Read the model definition and answer for the solid it produces. Units are mm, in the model's axes. Face numbers are marked on the shaded views. A direction names the side the tool comes from. Give positions to 0.01 mm unless a question says otherwise; leave off trailing zeros. Order: outer loops, then holes, each group sorted by start corner. A loop starts at its lowest first (then second) coordinate and runs counter-clockwise, first axis right, second up. Notation, with made-up numbers: M 50,66.5 L 103,66.5 A5 ccw 103,71.5 Z; hole C 54,74.5 d2. An arc over 180 degrees is marked long. One line per item, written item: value.
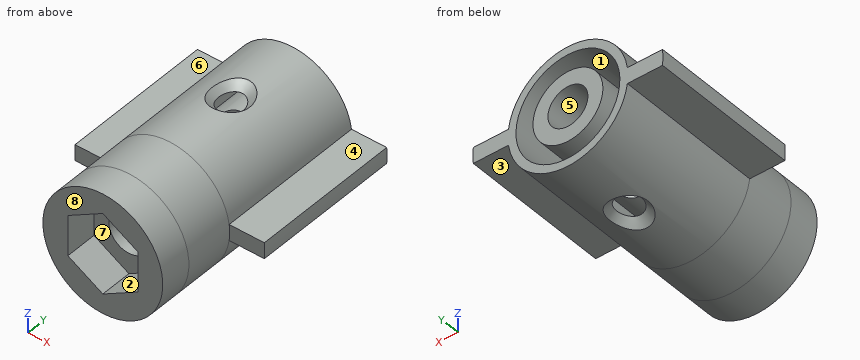
from build123d import *

# Parameters (mm, degrees)
SKETCH1_R           = 3.5
SKETCH1_R_2         = 2
BOSS_EXTRUDE1_DEPTH = 20
SKETCH1_3_R         = 6
BOSS_EXTRUDE2_DEPTH = 3.2
SKETCH1_4_R         = 6
BOSS_EXTRUDE3_DEPTH = 5
SKETCH2_R           = 5.2
BOSS_EXTRUDE4_DEPTH = 15
CIRPATTERN1_COUNT   = 2


with BuildPart() as part:
    # Sketch1 → Boss-Extrude1 (new body)
    with BuildSketch(Plane(origin=(0, 0, 0), x_dir=(1, 0, 0), z_dir=(0, 1, 0))):
        with Locations(Location((0, 0, 0), (0, 0, 270))):
            Circle(SKETCH1_R)
        with Locations(Location((0, 0, 0), (0, 0, 270))):
            Circle(SKETCH1_R_2, mode=Mode.SUBTRACT)
    extrude(amount=BOSS_EXTRUDE1_DEPTH)



with BuildPart() as body_2:
    # Sketch1_3 → Boss-Extrude2 (new body)
    with BuildSketch(Plane(origin=(0, 0, 0), x_dir=(1, 0, 0), z_dir=(0, 1, 0))):
        with Locations(Location((0, 0, 0), (0, 0, 270))):
            Circle(SKETCH1_3_R)
        Polygon((0, -4.041451884), (3.5, -2.020725942), (3.5, 2.020725942), (0, 4.041451884), (-3.5, 2.020725942), (-3.5, -2.020725942), align=None, mode=Mode.SUBTRACT)
    extrude(amount=-BOSS_EXTRUDE2_DEPTH)


with BuildPart() as part_1:
    add(part.part)

    add(body_2.part)  # Boss-Extrude3 merges body 2
    # Sketch1_4 → Boss-Extrude3 (add)
    # profile 1 of 7: a face of its own
    with BuildSketch(Plane(origin=(0, 0, 0), x_dir=(1, 0, 0), z_dir=(0, 1, 0))):
        with Locations(Location((0, 0, 0), (0, 0, 270))):
            Circle(SKETCH1_4_R)
        Polygon((0, -4.041451884), (3.5, -2.020725942), (3.5, 2.020725942), (0, 4.041451884), (-3.5, 2.020725942), (-3.5, -2.020725942), align=None, mode=Mode.SUBTRACT)
    # profile 2 of 7: a face of its own
    with BuildSketch(Plane(origin=(0, 0, 0), x_dir=(1, 0, 0), z_dir=(0, 1, 0))):
        with BuildLine():
            ThreePointArc((-1.749999906, 3.031088968), (8.8e-08, 3.5), (1.750000057, 3.03108888))
            Line((1.750000057, 3.03108888), (0, 4.041451884))
            Line((0, 4.041451884), (-1.749999906, 3.031088968))
        make_face()
    # profile 3 of 7: a face of its own
    with BuildSketch(Plane(origin=(0, 0, 0), x_dir=(1, 0, 0), z_dir=(0, 1, 0))):
        with BuildLine():
            ThreePointArc((1.750000057, 3.03108888), (3.03108893, 1.749999971), (3.5, 0))
            Line((3.5, 0), (3.5, 2.020725942))
            Line((3.5, 2.020725942), (1.750000057, 3.03108888))
        make_face()
    # profile 4 of 7: a face of its own
    with BuildSketch(Plane(origin=(0, 0, 0), x_dir=(1, 0, 0), z_dir=(0, 1, 0))):
        with BuildLine():
            Line((1.750000074, -3.03108887), (3.5, -2.020725942))
            Line((3.5, -2.020725942), (3.5, 0))
            ThreePointArc((3.5, 0), (3.031088935, -1.749999963), (1.750000074, -3.03108887))
        make_face()
    # profile 5 of 7: a face of its own
    with BuildSketch(Plane(origin=(0, 0, 0), x_dir=(1, 0, 0), z_dir=(0, 1, 0))):
        with BuildLine():
            Line((0, -4.041451884), (1.750000074, -3.03108887))
            ThreePointArc((1.750000074, -3.03108887), (5.1e-08, -3.5), (-1.749999986, -3.031088921))
            Line((-1.749999986, -3.031088921), (0, -4.041451884))
        make_face()
    # profile 6 of 7: a face of its own
    with BuildSketch(Plane(origin=(0, 0, 0), x_dir=(1, 0, 0), z_dir=(0, 1, 0))):
        with BuildLine():
            Line((-3.5, -2.020725942), (-1.749999986, -3.031088921))
            ThreePointArc((-1.749999986, -3.031088921), (-3.031088909, -1.750000007), (-3.5, 0))
            Line((-3.5, 0), (-3.5, -2.020725942))
        make_face()
    # profile 7 of 7: a face of its own
    with BuildSketch(Plane(origin=(0, 0, 0), x_dir=(1, 0, 0), z_dir=(0, 1, 0))):
        with BuildLine():
            ThreePointArc((-3.5, 0), (-3.031088886, 1.750000047), (-1.749999906, 3.031088968))
            Line((-1.749999906, 3.031088968), (-3.5, 2.020725942))
            Line((-3.5, 2.020725942), (-3.5, 0))
        make_face()
    extrude(amount=BOSS_EXTRUDE3_DEPTH)

    # Sketch2 → Boss-Extrude4 (add)
    with BuildSketch(Plane(origin=(0, 5, 0), x_dir=(1, 0, 0), z_dir=(0, 1, 0))):
        with BuildLine():
            Line((-9.46625586, -0.8), (-5.946427499, -0.8))
            ThreePointArc((-5.946427499, -0.8), (0, -6), (5.946427499, -0.8))
            Line((5.946427499, -0.8), (9.46625586, -0.8))
            ThreePointArc((9.46625586, -0.8), (9.5, 0), (9.46625586, 0.8))
            Line((9.46625586, 0.8), (5.946427499, 0.8))
            ThreePointArc((5.946427499, 0.8), (0, 6), (-5.946427499, 0.8))
            Line((-5.946427499, 0.8), (-9.46625586, 0.8))
            ThreePointArc((-9.46625586, 0.8), (-9.5, 0), (-9.46625586, -0.8))
        make_face()
        with Locations(Location((0, 0, 0), (0, 0, 270))):
            Circle(SKETCH2_R, mode=Mode.SUBTRACT)
    extrude(amount=BOSS_EXTRUDE4_DEPTH)

    # Sketch5 → CSK for M2 Flat Head Machine Screw1 (revolve, cut)
    with BuildSketch(Plane(origin=(0, 12.5, -6), x_dir=(0, 1, 0), z_dir=(1, 0, 0))):
        Polygon((0, 0), (0, 5), (1.2, 4.278967257), (1.2, 1), (2.2, 0), align=None)
    csk_for_m2_flat_head_machine_screw1 = revolve(axis=Axis((0, 12.5, -12.35), (0, 0, 1)), mode=Mode.SUBTRACT)

    # CirPattern1: CSK for M2 Flat Head Machine Screw1 ×2 about axis
    cirpattern1_axis = Axis((0, 5, 0), (0, -1, 0))
    for i in range(1, CIRPATTERN1_COUNT):
        add(csk_for_m2_flat_head_machine_screw1.rotate(cirpattern1_axis, i * 360 / CIRPATTERN1_COUNT), mode=Mode.SUBTRACT)


solid = part_1.part
1) Find section D-D, the plane z = -4.5. Write down the section's boundary in (x, y), plus the area to 3 significant figures.
Reported:
outline: M -3.97,-3.2 L 3.97,-3.2 L 3.97,20 L 2.61,20 L 2.61,5 L -2.61,5 L -2.61,20 L -3.97,20 Z
area: 106 mm^2
2) Find section C-C, the plane y = 12.5. Write down the section's boundary in (x, z).
Reported:
outline: M -9.47,-0.8 L -5.95,-0.8 A6 ccw -1.89,-5.69 L -1.25,-5.05 A5.2 cw -1.25,5.05 L -1.89,5.69 A6 ccw -5.95,0.8 L -9.47,0.8 A9.5 ccw Z; M -1.2,-3.29 L -1.2,-1.72 L -1.11,-1.67 A2 cw -1.11,1.67 L -1.2,1.72 L -1.2,3.29 A3.5 ccw Z; M 1.11,-1.67 L 1.2,-1.72 L 1.2,-3.29 A3.5 ccw 1.2,3.29 L 1.2,1.72 L 1.11,1.67 A2 cw Z; M 1.25,-5.05 L 1.89,-5.69 A6 ccw 5.95,-0.8 L 9.47,-0.8 A9.5 ccw 9.47,0.8 L 5.95,0.8 A6 ccw 1.89,5.69 L 1.25,5.05 A5.2 cw Z
3) Each of these flat-tipped pins is pushed along its axis until it touches: pin 1 Ø1.8 at (x, y) = (-8, 13.5) entering from -Z; pin 2 Ø2.5 at (y, z) = (-2, 0) entering from -X; pin 3 Ø1.8 at (x, y) = (-7.5, 12.5) entering from +Z; pin 4 Ø2 at (x, y) = (0, 12.5) entering from -Z. Where does it stop, or does it pass through?
Reported:
pin 1: stops at z = -0.8
pin 2: stops at x = -6
pin 3: stops at z = 0.8
pin 4: passes through
4) Consider probe 1 along Z at (x, y) = (0, 4.5); probe 2 along X at (y, z) = (12.5, 2.4); probe 3 along X at (y, z) = (12.5, -2.35). Determine where each line is inside the solid, lowest interval first.
Reported:
probe 1: z = -6 to -2, 2 to 6
probe 2: x = -5.5 to -4.61, -2.55 to -1.2, 1.2 to 2.55, 4.61 to 5.5
probe 3: x = -5.52 to -4.64, -2.59 to -1.2, 1.2 to 2.59, 4.64 to 5.52
5) Determine the mould class of the marked faces 5, 6, 7 and 8 for opening direction Z: +Z half, -Z half, draft (parallel to the pull), parting line (faces both ways), or undercut.
Reported:
face 5: undercut
face 6: +Z half
face 7: undercut
face 8: draft
6) Which of the six approach directions +Z, -Z, +X, -X, +Y, -Y give full straight-line access (tool end or side, diameter ignored) to the marked faces 1, 2, 3 and 4?
Reported:
face 1: +Y
face 2: -Y
face 3: -Z, +X, +Y, -Y
face 4: +Z, +X, +Y, -Y
7) Find section A-A, the plane y = 15.5. Write down the section's boundary in (x, z).
Reported:
outline: M -9.47,-0.8 L -5.95,-0.8 A6 ccw 5.95,-0.8 L 9.47,-0.8 A9.5 ccw 9.47,0.8 L 5.95,0.8 A6 ccw -5.95,0.8 L -9.47,0.8 A9.5 ccw Z; C 0,0 d7; hole C 0,0 d10.4; hole C 0,0 d4
8) Find section B-B, the plane z = 0. Write down the section's boundary in (x, y), plus the area to 3 significant figures.
Reported:
outline: M -9.5,5 L -6,5 L -6,-3.2 L -3.5,-3.2 L -3.5,0 L -2,0 L -2,20 L -3.5,20 L -3.5,5 L -5.2,5 L -5.2,20 L -9.5,20 Z; M 2,0 L 3.5,0 L 3.5,-3.2 L 6,-3.2 L 6,5 L 9.5,5 L 9.5,20 L 5.2,20 L 5.2,5 L 3.5,5 L 3.5,20 L 2,20 Z
area: 230 mm^2
